```python
from build123d import *

# Parameters (mm, degrees)
BOSS_EXTRUDE1_DEPTH = 6.35
FILLET1_R           = 8.255
SKETCH2_R           = 3.175
CUT_EXTRUDE1_DEPTH  = 128.158650905
CHAMFER2_START      = -126.7457463
CHAMFER2_OUTLINE_W  = 36
CHAMFER2_OUTLINE_H  = 6.35
CHAMFER2_DEPTH      = 83.771913248
FILLET4_R           = 20.955
FILLET5_R           = 12.7
SKETCH3_W           = 25.4
SKETCH3_H           = 25.4
SKETCH3_R           = 3.175
BOSS_EXTRUDE2_DEPTH = 6.35
SKETCH4_W           = 25.4
SKETCH4_H           = 177.8
SKETCH4_R           = 3.175
BOSS_EXTRUDE3_DEPTH = 6.35
SKETCH5_W           = 25.4
SKETCH5_H           = 101.6
CUT_EXTRUDE2_DEPTH  = 144.824345992
CHAMFER3_DEPTH      = 6.35
FILLET7_R           = 22.86
SKETCH6_R           = 2.38125
CUT_EXTRUDE3_DEPTH  = 144.824345992


with BuildPart() as part:
    # Sketch1 → Boss-Extrude1 (new body)
    with BuildSketch(Plane.XY):
        with BuildLine():
            Line((12.7, 76.2), (-12.7, 76.2))
            Line((-12.7, 76.2), (-12.7, -28.680951188))
            ThreePointArc((-12.7, -28.680951188), (-71.390768363, -25.798437524), (-101.6, -76.2))
            Line((-101.6, -76.2), (-85.725, -76.2))
            ThreePointArc((-85.725, -76.2), (-58.470420375, -37.379213847), (-12.7, -49.826469235))
            Line((-12.7, -49.826469235), (-12.7, -76.2))
            Line((-12.7, -76.2), (12.7, -76.2))
            Line((12.7, -76.2), (12.7, 76.2))
        make_face()
    extrude(amount=BOSS_EXTRUDE1_DEPTH)

    # Fillet1
    fillet1_edges = [part.edges().sort_by_distance(p)[0] for p in [
        (-12.7, -49.826469235, 3.175),
    ]]
    fillet(fillet1_edges, radius=FILLET1_R)

    # Chamfer1
    # the kernel refuses this chamfer: 16.925734726, 15.24 mm, written as the material it takes off along each edge
    with BuildSketch(Plane(origin=(-85.725, -76.2, -32.922584323), x_dir=(0.15149402541241913, 0.9884581732498049, 0), z_dir=(0, 0, 1))) as chamfer1_piece_1:
        with BuildLine():
            Line((13.017434015, -0.44343203), (-2.4273823, 12.943386903))
            Line((-2.4273823, 12.943386903), (-2.761989917, 12.89210395))
            ThreePointArc((-2.761989917, 12.89210395), (-1.331569383, 6.453627085), (-0.334607617, -0.051282954))
            Line((-0.334607617, -0.051282954), (0.051282954, -0.334607617))
            ThreePointArc((0.051282954, -0.334607617), (6.510978775, 0.137060785), (12.966151061, -0.778039646))
            Line((12.966151061, -0.778039646), (13.017434015, -0.44343203))
        make_face()
    extrude(amount=72.195168646, mode=Mode.SUBTRACT)

    # Sketch2 → Cut-Extrude1 (cut, through all)
    with BuildSketch(Plane.XY.offset(6.35)):
        with Locations((0, 57.15)):
            Circle(SKETCH2_R)
        with Locations((0, 69.85)):
            Circle(SKETCH2_R)
    extrude(amount=-CUT_EXTRUDE1_DEPTH, mode=Mode.SUBTRACT)

    # Chamfer2: read off the stored shape, not the designer's step
    # Chamfer2 outline → Chamfer2 (cut)
    with BuildSketch(Plane(origin=(0, 0, 0), x_dir=(0.6493951635681026, -0.7604511302735748, 0), z_dir=(0.7604511302735747, 0.6493951635681027, 0)).offset(CHAMFER2_START)):
        with Locations((47, -3.175)):
            Rectangle(CHAMFER2_OUTLINE_W, CHAMFER2_OUTLINE_H)
    extrude(amount=CHAMFER2_DEPTH, mode=Mode.SUBTRACT)

    # Fillet4
    # the kernel refuses this fillet: 20.955 mm, written as the material it takes off along each edge
    with BuildSketch(Plane(origin=(8.560811014, -76.2, 27.244649936), x_dir=(1, 0, 0), z_dir=(0, 0, -1))) as fillet4_piece_1:
        with BuildLine():
            CenterArc((10.50769959, -19.963819717), FILLET4_R, 107.692818626, 31.811166067)
            Line((-5.427553845, -6.355744064), (-5.746258914, -6.083582551))
            Line((-5.746258914, -6.083582551), (-0.318705069, 0.272161513))
            Line((-0.318705069, 0.272161513), (0, 0.4191))
            ThreePointArc((0, 0.4191), (2.069594493, 0.4191), (4.011818774, 0.399276394))
            Line((4.011818774, 0.399276394), (4.139188986, 0))
        make_face()
    extrude(amount=48.139299873, mode=Mode.SUBTRACT)

    # Fillet5
    fillet5_edges = [part.edges().sort_by_distance(p)[0] for p in [
        (-12.7, -28.680951188, 3.175),
    ]]
    fillet(fillet5_edges, radius=FILLET5_R)

    # Sketch3 → Boss-Extrude2 (add)
    with BuildSketch(Plane.XY.offset(6.35)):
        with Locations((0, 88.9)):
            Rectangle(SKETCH3_W, SKETCH3_H)
        with Locations((0, 95.25)):
            Circle(SKETCH3_R, mode=Mode.SUBTRACT)
    extrude(amount=-BOSS_EXTRUDE2_DEPTH)

    # Sketch4 → Boss-Extrude3 (add)
    with BuildSketch(Plane(origin=(0, 0, 0), x_dir=(-1, 0, 0), z_dir=(0, 0, -1))):
        with Locations((-25.4, 12.7)):
            Rectangle(SKETCH4_W, SKETCH4_H)
        with Locations((-25.4, 95.25)):
            Circle(SKETCH4_R, mode=Mode.SUBTRACT)
        with Locations((-25.4, 69.85)):
            Circle(SKETCH4_R, mode=Mode.SUBTRACT)
        with Locations((-25.4, 57.15)):
            Circle(SKETCH4_R, mode=Mode.SUBTRACT)
    extrude(amount=-BOSS_EXTRUDE3_DEPTH)

    # Sketch5 → Cut-Extrude2 (cut, through all)
    with BuildSketch(Plane(origin=(0, 0, 0), x_dir=(-1, 0, 0), z_dir=(0, 0, -1))):
        with Locations((0, 50.8)):
            Rectangle(SKETCH5_W, SKETCH5_H)
    extrude(amount=-CUT_EXTRUDE2_DEPTH, mode=Mode.SUBTRACT)

    # Chamfer3: read off the stored shape, not the designer's step
    # Chamfer3 outline → Chamfer3 (cut)
    with BuildSketch(Plane.XY):
        with BuildLine():
            ThreePointArc((-12.7, -8.997916699), (-13.235467867, -12.646773779), (-14.796717794, -15.98793862))
            Line((-14.796717794, -15.98793862), (12.7, -1.180669249))
            Line((12.7, -1.180669249), (12.7, 0))
            Line((12.7, 0), (-12.7, 0))
            Line((-12.7, 0), (-12.7, -8.997916699))
        make_face()
    extrude(amount=CHAMFER3_DEPTH, mode=Mode.SUBTRACT)

    # Fillet7
    fillet7_edges = [part.edges().sort_by_distance(p)[0] for p in [
        (-14.796717794, -15.98793862, 3.175),
        (12.7, -1.180669249, 3.175),
    ]]
    fillet(fillet7_edges, radius=FILLET7_R)

    # Sketch6 → Cut-Extrude3 (cut, through all)
    with BuildSketch(Plane(origin=(0, 0, 0), x_dir=(-1, 0, 0), z_dir=(0, 0, -1))):
        with Locations((89.842397197, -57.554736727)):
            Circle(SKETCH6_R)
        with Locations((75.517874882, -38.214440689)):
            Circle(SKETCH6_R)
        with Locations((52.406792333, -27.776813182)):
            Circle(SKETCH6_R)
        with Locations((27.741530006, -30.059534069)):
            Circle(SKETCH6_R)
    extrude(amount=-CUT_EXTRUDE3_DEPTH, mode=Mode.SUBTRACT)


solid = part.part
```
Can you work these out from the model? Positions are in its coordinate system, mm. A direction names the side the tool comes from. Round coordinates to 2 decimals unless told otherwise and drop trailing zeros. Loops run counter-clockwise (first coordinate to the right, second up) from the corner with the lowest first, then second, coordinate; pieces in that order, holes last.
Item 1: Suppose I cut it at B-B, the plane x = 25.4. Write out the boundary of the cut face in (y, z) (3 decimals), then the cut area to 3 significant figures.
Item 2: Suppose I cut it at C-C, the plane z = 3. State how many separate pieces and enclosed holes the cut face has, then the cut area to 3 significant figures.
Item 3: Please list where these lines run through material, in increasing order: L1, parallel to Y at x = 25.4, z = 3.75 (3 decimals); L2, parallel to Y at x = 27, z = 0.5; L3, parallel to X at y = 75.5, z = 3.5.
Item 4: If we mould it in two halves opening along Y, with no side actions, what happens to faces 3 (the flat face through (12.7, 56, 3)), 4 (the cylindrical face through (-78.32, -30.17, 3.13)), 5 (the cylindrical face through (-92.04, -58.47, 3.13))? For each: +Y half, -Y half, draft (parallel to the pull), parting line (faces both ways), or undercut.
Item 5: Suppose I cut it at A-A, the plane y = 57.15. Write out the boundary of the cut face in (x, z) (3 decimals), then the cut area to 3 significant figures.
Item 6: Suppose I cut it at D-D, the plane y = 37. Write out the boundary of the cut face in (x, z), then the cut area to 3 significant figures.
Item 7: Which directions (+Z, -Z, +X, -X, +Y, -Y) give clear straight access to the entire face, cutting with the end or side of a thin tool? Please do faces 1 (the cylindrical face through (9.554, 0.899, 3.219)), 2 (the flat face through (-5.016, -60.301, 3.131)).
Item 8: Will this pin go through, and if not, where does the flat tip stop? pin 1 Ø1.5 at (x, z) = (-13, 5) entering from +Y.
Reported:
1. outline: (-76.2, 0) - (53.975, 0) - (53.975, 6.35) - (-76.2, 6.35) - close; (60.325, 0) - (66.675, 0) - (66.675, 6.35) - (60.325, 6.35) - close; (73.025, 0) - (92.075, 0) - (92.075, 6.35) - (73.025, 6.35) - close; (98.425, 0) - (101.6, 0) - (101.6, 6.35) - (98.425, 6.35) - close
1. area: 1,010 mm2
2. separate pieces: 1
2. enclosed holes: 7
2. area: 7,620 mm2
3. L1: y = -76.2 to 53.975, 60.325 to 66.675, 73.025 to 92.075, 98.425 to 101.6
3. L2: y = -76.2 to 54.41, 59.89 to 67.11, 72.59 to 92.51, 97.99 to 101.6
3. L3: x = 12.7 to 38.1
4. face 3: draft
4. face 4: +Y half
4. face 5: undercut
5. outline: (12.7, 0) - (22.225, 0) - (22.225, 6.35) - (12.7, 6.35) - close; (28.575, 0) - (38.1, 0) - (38.1, 6.35) - (28.575, 6.35) - close
5. area: 121 mm2
6. outline: (12.7, 0) - (38.1, 0) - (38.1, 6.35) - (12.7, 6.35) - close
6. area: 161 mm2
7. face 1: +Z, -Z, -X, +Y
7. face 2: +Z, -Z, -Y
8. pin 1: stops at y = -14.66
